Autodesk Inventor part; units mm, degrees
ref_plane "YZ Plane" through (0, 0, 0) normal (1, 0, 0) x (0, 1, 0)
ref_plane "XZ Plane" through (0, 0, 0) normal (0, 1, 0) x (-1, 0, 0)
ref_plane "XY Plane" through (0, 0, 0) normal (0, 0, 1) x (1, 0, 0)
sketch "Sketch4" plane through (0, 0, 0) normal (0, 0, 1) x (1, 0, 0)
  line L0 (-28.9374, -10.0235) -> (-36.7376, -0.0011)
  line L1 (-28.9374, -10.0235) -> (-16.2374, -10.0235) construction
  line L2 (-36.7376, -0.0011) -> (-15.7934, 29.7213)
  line L3 (-15.7934, 29.7213) -> (-28.9374, -10.0235)
  line L4 (0, 0) -> (0, 43.134) construction
  line L5 (0, -17.5109) -> (-45.4613, -17.5109) construction
  line L6 (-45.4613, -17.5109) -> (54.0034, -17.5109) construction
  line L7 (28.9374, -10.0235) -> (36.7376, -0.0011)
  line L8 (36.7376, -0.0011) -> (15.7934, 29.7213)
  line L9 (15.7934, 29.7213) -> (28.9374, -10.0235)
  line L10 (-28.9374, -24.9984) -> (-36.7376, -35.0207)
  line L11 (-36.7376, -35.0207) -> (-15.7934, -64.7432)
  line L12 (-15.7934, -64.7432) -> (-28.9374, -24.9984)
  line L13 (15.7934, -64.7432) -> (28.9374, -24.9984)
  line L14 (36.7376, -35.0207) -> (15.7934, -64.7432)
  line L15 (28.9374, -24.9984) -> (36.7376, -35.0207)
  dimension "d9" = 12.7
sketch "Sketch5" plane through (0, 0, 0) normal (0, 0, 1) x (1, 0, 0)
  line L0 (-58.3358, 40.999) -> (58.3358, 40.999)
  line L1 (58.3358, 40.999) -> (58.3358, -76.1205)
  line L2 (58.3358, -76.1205) -> (-58.3358, -76.1205)
  line L3 (-58.3358, -76.1205) -> (-58.3358, 40.999)
  line L4 (-58.3358, 40.999) -> (58.3358, -76.1205) construction
  line L5 (58.3358, 40.999) -> (-58.3358, -76.1205) construction
  point P0 (0, 0)
  point P1 (0, -17.5607)
extrude "Extrusion4" add sketch "Sketch4" against normal blind 25.4
extrude "Extrusion5" add sketch "Sketch5" against normal blind 12.7
sketch "Sketch6" plane through (0, 0, -12.7) normal (0, 0, -1) x (-1, 0, 0)
  line L0 (-23.8244, -6.5433) -> (-21.2379, -6.5433)
  line L1 (-20.9936, 4.8166) -> (-6.9933, 4.8166)
  line L2 (-6.9933, 4.8166) -> (0, -43.0842)
  line L3 (0, -43.0842) -> (8.4371, 5.9599)
  line L4 (8.4371, 5.9599) -> (21.8678, 5.9599)
  line L5 (21.8678, 5.9599) -> (0, -59.2796)
  line L6 (0, -59.2796) -> (-20.9936, 4.8166)
  point P0 (0, 0)
extrude "Extrusion6" add sketch "Sketch6" along normal blind 12.7
sketch "Sketch7" plane through (0, 0, -12.7) normal (0, 0, -1) x (-1, 0, 0)
  line L0 (-19.319, 35.5552) -> (28.0582, 35.5552) construction
  line L1 (28.0582, 35.5552) -> (28.0582, 31.6649) construction
  line L2 (28.0582, 31.6649) -> (-19.319, 31.6649) construction
  line L3 (-19.319, 31.6649) -> (-19.319, 35.5552) construction
  point P0 (0, 0)
properties part number "Logo"
Geometry: final body of the model. Coordinates: model frame, mm. A direction names the side the tool comes from. Coordinates: 2 decimals unless noted, no trailing zeros. Order: outer loops, then holes, each group sorted by start corner. A loop starts at its lowest first (then second) coordinate and runs counter-clockwise, first axis right, second up. Notation, with made-up numbers: (9, -20) - (63, -20) arc R23 ccw to (63, -5) - close; hole circle Ø9 at (5, -4.5). An arc over 180 degrees is marked (long way). Use one line per item in the form item = value.
1) Ray query, L1, parallel to Z at x = -3, y = -65.5; L2, parallel to X at y = -24, z = -22.75; L3, parallel to X at y = 18.5, z = -14. Return the intervals inside material, ascending.
Solutions:
L1 = -12.7 to 0
L2 = -11.83 to -3.28, 2.79 to 11.56
L3 = -23.7 to -19.5, 19.5 to 23.7
2) Mould query, pull axis Y, two halves, no side actions, for faces 1 (the face through (-32.783, -29.939, -18.961)), 2 (the face through (-1, 40.999, -6)), 3 (the face through (-58.336, -18, -6)). Classes: +Y half, -Y half, draft (parallel to the pull), parting line (faces both ways), or undercut.
Solutions:
face_1 = undercut
face_2 = +Y half
face_3 = draft
3) Section A-A (z = -20). Return loops of the section in (x, y), then the cut area to 3 significant figures.
Solutions:
outline = (-36.74, -35.02) - (-15.79, -64.74) - (-28.94, -25) - close; (-36.74, 0) - (-28.94, -10.02) - (-15.79, 29.72) - close; (-21.87, 5.96) - (0, -59.28) - (20.99, 4.82) - (6.99, 4.82) - (0, -43.08) - (-8.44, 5.96) - close; (15.79, -64.74) - (36.74, -35.02) - (28.94, -25) - close; (15.79, 29.72) - (28.94, -10.02) - (36.74, 0) - close
area = 1,900 mm^2
4) Section D-D (y = 9). Return loops of the section in (x, z), then the cut area to 3 significant figures.
Solutions:
outline = (-58.34, -12.7) - (-30.39, -12.7) - (-30.39, -25.4) - (-22.65, -25.4) - (-22.65, -12.7) - (22.65, -12.7) - (22.65, -25.4) - (30.39, -25.4) - (30.39, -12.7) - (58.34, -12.7) - (58.34, 0) - (-58.34, 0) - close
area = 1,680 mm^2
5) Section C-C (y = -51.5). Return loops of the section in (x, z).
Solutions:
outline = (-58.34, -12.7) - (-25.13, -12.7) - (-25.13, -25.4) - (-20.17, -25.4) - (-20.17, -12.7) - (-2.61, -12.7) - (-2.61, -25.4) - (2.55, -25.4) - (2.55, -12.7) - (20.17, -12.7) - (20.17, -25.4) - (25.13, -25.4) - (25.13, -12.7) - (58.34, -12.7) - (58.34, 0) - (-58.34, 0) - close
6) Pin query (flat end, axial travel): pin 1 (4 mm diameter, centred on x = -18, z = -17.5, fed in from +Y); pin 2 (4 mm diameter, centred on x = 17, z = -21.5, fed in from +Y); pin 3 (3 mm diameter, centred on x = 23, y = 29, fed in from -Z); pin 4 (6 mm diameter, centred on y = -39, z = -13, fed in from -X). Return the tip coordinate at first contact, or that it passes through.
Solutions:
pin_1 = 29.43
pin_2 = 29.72
pin_3 = -12.7
pin_4 = -58.34
7) Set-up query: faces 4 (the face through (32.783, -5.082, -18.961)), 5 (the face through (-4.16, -18.91, -18.96)), 6 (the face through (-26.412, -49.674, -18.961)), 7 (the face through (-11.09, -26.2, -18.96)). Return all of +Z, -Z, +X, -X, +Y, -Y with unobstructed straight access to the full face (end or side cutting, diameter ignored); none if empty.
Solutions:
face_4 = -Z, +X
face_5 = -Z, +Y
face_6 = -Z, -X, -Y
face_7 = -Z
8) Section B-B (x = 26). Return loops of the section in (y, z), then the cut area to 3 significant figures.
Solutions:
outline = (-76.12, -12.7) - (-50.26, -12.7) - (-50.26, -25.4) - (-33.88, -25.4) - (-33.88, -12.7) - (-1.14, -12.7) - (-1.14, -25.4) - (15.24, -25.4) - (15.24, -12.7) - (41, -12.7) - (41, 0) - (-76.12, 0) - close
area = 1,900 mm^2
